Geometry: final body of the model. Coordinates: model frame, mm. Face numbers are marked on the shaded views. A direction names the side the tool comes from. Give positions to 0.01 mm unless a question says otherwise; leave off trailing zeros. Loops run counter-clockwise (first coordinate to the right, second up) from the corner with the lowest first, then second, coordinate; pieces in that order, holes last. Notation, with made-up numbers: M 76,69.25 L 84,69.25 A17 cw 84,88.25 Z; hole C 53,67 d5. An arc over 180 degrees is marked long. One line per question, with ' | ' between items. Start each with the question number.
from build123d import *

# Parameters (mm, degrees)
BOSS_EXTRUDE1_DEPTH            = 294.64
SKETCH3_W                      = 68.7
SKETCH3_H                      = 6.35
BOSS_EXTRUDE2_DEPTH            = 48
CUT_EXTRUDE2_REACH             = 304.363
SKETCH4_R                      = 1.3890625
SKETCH4_R_2                    = 11
SKETCH4_W                      = 26
SKETCH4_H                      = 72
CUT_EXTRUDE3_REACH             = 303.286
SKETCH5_R                      = 1.7859375
CUT_EXTRUDE4_REACH             = 309.814
SKETCH6_R                      = 1.3890625
CUT_EXTRUDE4_DIRECTION_2_REACH = 309.814
CUT_EXTRUDE5_REACH             = 309.814
SKETCH11_R                     = 0.889
SKETCH12_W                     = 68.7
SKETCH12_H                     = 6.35
CUT_EXTRUDE6_DEPTH             = 50.8
BOSS_EXTRUDE3_DEPTH            = 50
SKETCH14_W                     = 81.4
SKETCH14_H                     = 54.35
BOSS_EXTRUDE4_DEPTH            = 6.35
SKETCH15_W                     = 68.7
SKETCH15_H                     = 50
BOSS_EXTRUDE5_DEPTH            = 1
SKETCH16_W                     = 190.5
SKETCH16_H                     = 19.05
CUT_EXTRUDE7_DEPTH             = 4.175
SKETCH17_W                     = 190.5
SKETCH17_H                     = 19.05
CUT_EXTRUDE8_DEPTH             = 4.175
CUT_EXTRUDE9_DEPTH             = 310.015097083
CUT_EXTRUDE9_DEPTH_BACK        = 310.015097083
SKETCH18_R                     = 0.889


with BuildPart() as part:
    # Sketch1 → Boss-Extrude1 (new body)
    with BuildSketch(Plane.XY):
        Polygon((0, 0), (34.35, 0), (34.35, 48), (40.7, 48), (40.7, -6.35), (0, -6.35), align=None)
    extrude(amount=BOSS_EXTRUDE1_DEPTH)

    # Mirror1: part across plane


with BuildPart() as part_1:
    add(part.part)
    add(part.part.mirror(Plane(origin=(0, -6.35, 294.64), x_dir=(0, 0, 1), z_dir=(1, 0, 0))))

    # Sketch3 → Boss-Extrude2 (add)
    with BuildSketch(Plane(origin=(0, 0, 0), x_dir=(1, 0, 0), z_dir=(0, 1, 0))):
        with Locations((0, -3.175)):
            Rectangle(SKETCH3_W, SKETCH3_H)
    extrude(amount=BOSS_EXTRUDE2_DEPTH)

    # Sketch4 → Cut-Extrude2 (cut, up to next)
    with BuildSketch(Plane.XZ.offset(6.35), mode=Mode.PRIVATE) as cut_extrude2_sk1:
        with Locations((0, 12.7)):
            Circle(SKETCH4_R)
    cut_extrude2_tool1 = extrude(cut_extrude2_sk1.sketch, amount=-CUT_EXTRUDE2_REACH, mode=Mode.PRIVATE) & part_1.part
    # Sketch4 → Cut-Extrude2 (cut, up to next)
    with BuildSketch(Plane.XZ.offset(6.35), mode=Mode.PRIVATE) as cut_extrude2_sk2:
        with Locations((0, 95.2)):
            Circle(SKETCH4_R)
    cut_extrude2_tool2 = extrude(cut_extrude2_sk2.sketch, amount=-CUT_EXTRUDE2_REACH, mode=Mode.PRIVATE) & part_1.part
    # Sketch4 → Cut-Extrude2 (cut, up to next)
    with BuildSketch(Plane.XZ.offset(6.35), mode=Mode.PRIVATE) as cut_extrude2_sk3:
        with Locations((0, 53.95)):
            Circle(SKETCH4_R_2)
    cut_extrude2_tool3 = extrude(cut_extrude2_sk3.sketch, amount=-CUT_EXTRUDE2_REACH, mode=Mode.PRIVATE) & part_1.part
    # Sketch4 → Cut-Extrude2 (cut, up to next)
    with BuildSketch(Plane.XZ.offset(6.35), mode=Mode.PRIVATE) as cut_extrude2_sk4:
        with Locations((-3.2622, 160.64)):
            Rectangle(SKETCH4_W, SKETCH4_H)
    cut_extrude2_tool4 = extrude(cut_extrude2_sk4.sketch, amount=-CUT_EXTRUDE2_REACH, mode=Mode.PRIVATE) & part_1.part
    add(cut_extrude2_tool1.solids().sort_by_distance((0, -6.35, 12.7))[0], mode=Mode.SUBTRACT)
    add(cut_extrude2_tool2.solids().sort_by_distance((0, -6.35, 95.2))[0], mode=Mode.SUBTRACT)
    add(cut_extrude2_tool3.solids().sort_by_distance((0, -6.35, 53.95))[0], mode=Mode.SUBTRACT)
    add(cut_extrude2_tool4.solids().sort_by_distance((-3.2622, -6.35, 160.64))[0], mode=Mode.SUBTRACT)

    # Sketch5 → Cut-Extrude3 (cut, up to next)
    with BuildSketch(Plane(origin=(0, 0, 0), x_dir=(1, 0, 0), z_dir=(0, 1, 0)), mode=Mode.PRIVATE) as cut_extrude3_sk1:
        with Locations(Location((16.0628, -195.74, 0), (0, 0, 270))):
            Circle(SKETCH5_R)
    cut_extrude3_tool1 = extrude(cut_extrude3_sk1.sketch, amount=-CUT_EXTRUDE3_REACH, mode=Mode.PRIVATE) & part_1.part
    # Sketch5 → Cut-Extrude3 (cut, up to next)
    with BuildSketch(Plane(origin=(0, 0, 0), x_dir=(1, 0, 0), z_dir=(0, 1, 0)), mode=Mode.PRIVATE) as cut_extrude3_sk2:
        with Locations(Location((16.0628, -139.74, 0), (0, 0, 270))):
            Circle(SKETCH5_R)
    cut_extrude3_tool2 = extrude(cut_extrude3_sk2.sketch, amount=-CUT_EXTRUDE3_REACH, mode=Mode.PRIVATE) & part_1.part
    add(cut_extrude3_tool1.solids().sort_by_distance((16.0628, 0, 195.74))[0], mode=Mode.SUBTRACT)
    add(cut_extrude3_tool2.solids().sort_by_distance((16.0628, 0, 139.74))[0], mode=Mode.SUBTRACT)

    # Cut-Extrude4: up to this face of the body (flat: up to its plane)
    cut_extrude4_end = Plane(part_1.part.faces().sort_by_distance((40.7, 20.825, 147.32))[0])
    # Sketch6 → Cut-Extrude4 (cut, up to the picked face)
    with BuildSketch(Plane(origin=(-34.35, 0, 0), x_dir=(0, 0, -1), z_dir=(1, 0, 0)), mode=Mode.PRIVATE) as cut_extrude4_sk1:
        with Locations(Location((-287.14, 32.15, 0), (0, 0, 180))):
            Circle(SKETCH6_R)
    cut_extrude4_tool1 = split(extrude(cut_extrude4_sk1.sketch, amount=CUT_EXTRUDE4_REACH, mode=Mode.PRIVATE), bisect_by=cut_extrude4_end, keep=Keep.BOTH, mode=Mode.PRIVATE)
    # Sketch6 → Cut-Extrude4 (cut, up to the picked face)
    with BuildSketch(Plane(origin=(-34.35, 0, 0), x_dir=(0, 0, -1), z_dir=(1, 0, 0)), mode=Mode.PRIVATE) as cut_extrude4_sk2:
        with Locations(Location((-122.14, 32.15, 0), (0, 0, 180))):
            Circle(SKETCH6_R)
    cut_extrude4_tool2 = split(extrude(cut_extrude4_sk2.sketch, amount=CUT_EXTRUDE4_REACH, mode=Mode.PRIVATE), bisect_by=cut_extrude4_end, keep=Keep.BOTH, mode=Mode.PRIVATE)
    add(cut_extrude4_tool1.solids().sort_by(Axis((-34.35, 32.15, 287.14), (1, 0, 0)))[0], mode=Mode.SUBTRACT)
    add(cut_extrude4_tool2.solids().sort_by(Axis((-34.35, 32.15, 122.14), (1, 0, 0)))[0], mode=Mode.SUBTRACT)

    # Cut-Extrude4 direction 2: up to this face of the body (flat: up to its plane)
    cut_extrude4_direction_2_end = Plane(part_1.part.faces().sort_by_distance((-40.7, 20.825, 147.32))[0])
    # Sketch6 → Cut-Extrude4 direction 2 (cut, up to the picked face)
    with BuildSketch(Plane(origin=(-34.35, 0, 0), x_dir=(0, 0, -1), z_dir=(1, 0, 0)), mode=Mode.PRIVATE) as cut_extrude4_direction_2_sk1:
        with Locations(Location((-287.14, 32.15, 0), (0, 0, 180))):
            Circle(SKETCH6_R)
    cut_extrude4_direction_2_tool1 = split(extrude(cut_extrude4_direction_2_sk1.sketch, amount=-CUT_EXTRUDE4_DIRECTION_2_REACH, mode=Mode.PRIVATE), bisect_by=cut_extrude4_direction_2_end, keep=Keep.BOTH, mode=Mode.PRIVATE)
    # Sketch6 → Cut-Extrude4 direction 2 (cut, up to the picked face)
    with BuildSketch(Plane(origin=(-34.35, 0, 0), x_dir=(0, 0, -1), z_dir=(1, 0, 0)), mode=Mode.PRIVATE) as cut_extrude4_direction_2_sk2:
        with Locations(Location((-122.14, 32.15, 0), (0, 0, 180))):
            Circle(SKETCH6_R)
    cut_extrude4_direction_2_tool2 = split(extrude(cut_extrude4_direction_2_sk2.sketch, amount=-CUT_EXTRUDE4_DIRECTION_2_REACH, mode=Mode.PRIVATE), bisect_by=cut_extrude4_direction_2_end, keep=Keep.BOTH, mode=Mode.PRIVATE)
    add(cut_extrude4_direction_2_tool1.solids().sort_by(Axis((-34.35, 32.15, 287.14), (-1, 0, 0)))[0], mode=Mode.SUBTRACT)
    add(cut_extrude4_direction_2_tool2.solids().sort_by(Axis((-34.35, 32.15, 122.14), (-1, 0, 0)))[0], mode=Mode.SUBTRACT)

    # Sketch11 → Cut-Extrude5 (cut, up to next)
    with BuildSketch(Plane.ZY.offset(-34.35), mode=Mode.PRIVATE) as cut_extrude5_sk1:
        with Locations((13.75, 5.5)):
            Circle(SKETCH11_R)
    cut_extrude5_tool1 = extrude(cut_extrude5_sk1.sketch, amount=-CUT_EXTRUDE5_REACH, mode=Mode.PRIVATE) & part_1.part
    # Sketch11 → Cut-Extrude5 (cut, up to next)
    with BuildSketch(Plane.ZY.offset(-34.35), mode=Mode.PRIVATE) as cut_extrude5_sk2:
        with Locations((13.75, 15)):
            Circle(SKETCH11_R)
    cut_extrude5_tool2 = extrude(cut_extrude5_sk2.sketch, amount=-CUT_EXTRUDE5_REACH, mode=Mode.PRIVATE) & part_1.part
    # Sketch11 → Cut-Extrude5 (cut, up to next)
    with BuildSketch(Plane.ZY.offset(-34.35), mode=Mode.PRIVATE) as cut_extrude5_sk3:
        with Locations((140.81, 15)):
            Circle(SKETCH11_R)
    cut_extrude5_tool3 = extrude(cut_extrude5_sk3.sketch, amount=-CUT_EXTRUDE5_REACH, mode=Mode.PRIVATE) & part_1.part
    # Sketch11 → Cut-Extrude5 (cut, up to next)
    with BuildSketch(Plane.ZY.offset(-34.35), mode=Mode.PRIVATE) as cut_extrude5_sk4:
        with Locations((140.81, 5.5)):
            Circle(SKETCH11_R)
    cut_extrude5_tool4 = extrude(cut_extrude5_sk4.sketch, amount=-CUT_EXTRUDE5_REACH, mode=Mode.PRIVATE) & part_1.part
    add(cut_extrude5_tool1.solids().sort_by_distance((34.35, 5.5, 13.75))[0], mode=Mode.SUBTRACT)
    add(cut_extrude5_tool2.solids().sort_by_distance((34.35, 15, 13.75))[0], mode=Mode.SUBTRACT)
    add(cut_extrude5_tool3.solids().sort_by_distance((34.35, 15, 140.81))[0], mode=Mode.SUBTRACT)
    add(cut_extrude5_tool4.solids().sort_by_distance((34.35, 5.5, 140.81))[0], mode=Mode.SUBTRACT)

    # Sketch12 → Cut-Extrude6 (cut)
    with BuildSketch(Plane.XY.offset(294.64)):
        with Locations((0, -3.175)):
            Rectangle(SKETCH12_W, SKETCH12_H)
    extrude(amount=-CUT_EXTRUDE6_DEPTH, mode=Mode.SUBTRACT)

    # Sketch13 → Boss-Extrude3 (add)
    with BuildSketch(Plane(origin=(0, 0, 0), x_dir=(-1, 0, 0), z_dir=(0, 0, -1))):
        Polygon((34.35, 48), (34.35, 0), (-34.35, 0), (-34.35, 48), (-40.7, 48), (-40.7, -6.35), (40.7, -6.35), (40.7, 48), align=None)
    extrude(amount=BOSS_EXTRUDE3_DEPTH)

    # Sketch14 → Boss-Extrude4 (add)
    with BuildSketch(Plane(origin=(0, 0, -50), x_dir=(-1, 0, 0), z_dir=(0, 0, -1))):
        with Locations((0, 20.825)):
            Rectangle(SKETCH14_W, SKETCH14_H)
    extrude(amount=BOSS_EXTRUDE4_DEPTH)

    # Sketch15 → Boss-Extrude5 (add)
    with BuildSketch(Plane(origin=(0, 48, 0), x_dir=(1, 0, 0), z_dir=(0, 1, 0))):
        Polygon((40.7, -294.64), (40.7, 56.35), (-40.7, 56.35), (-40.7, -294.64), (-34.35, -294.64), (-34.35, -6.35), (34.35, -6.35), (34.35, -294.64), align=None)
        with Locations((0, 25)):
            Rectangle(SKETCH15_W, SKETCH15_H, mode=Mode.SUBTRACT)
    extrude(amount=BOSS_EXTRUDE5_DEPTH)

    # Sketch16 → Cut-Extrude7 (cut)
    with BuildSketch(Plane(origin=(-34.35, 0, 0), x_dir=(0, 0, -1), z_dir=(1, 0, 0))):
        with Locations((-199.39, 32.15)):
            Rectangle(SKETCH16_W, SKETCH16_H)
    extrude(amount=-CUT_EXTRUDE7_DEPTH, mode=Mode.SUBTRACT)

    # Sketch17 → Cut-Extrude8 (cut)
    with BuildSketch(Plane.ZY.offset(-34.35)):
        with Locations((199.39, 32.15)):
            Rectangle(SKETCH17_W, SKETCH17_H)
    extrude(amount=-CUT_EXTRUDE8_DEPTH, mode=Mode.SUBTRACT)

    # Sketch18 → Cut-Extrude9 (cut, two sides: drawn at the far end of the back side and taken through both)
    with BuildSketch(Plane(origin=(-38.525, 0, 0), x_dir=(0, 0, -1), z_dir=(1, 0, 0)).offset(-CUT_EXTRUDE9_DEPTH_BACK)):
        with Locations((-287.14, 39.77)):
            Circle(SKETCH18_R)
        with Locations((-287.14, 24.53)):
            Circle(SKETCH18_R)
        with Locations((-122.14, 39.77)):
            Circle(SKETCH18_R)
        with Locations((-122.14, 24.53)):
            Circle(SKETCH18_R)
    extrude(amount=CUT_EXTRUDE9_DEPTH + CUT_EXTRUDE9_DEPTH_BACK, mode=Mode.SUBTRACT)


solid = part_1.part
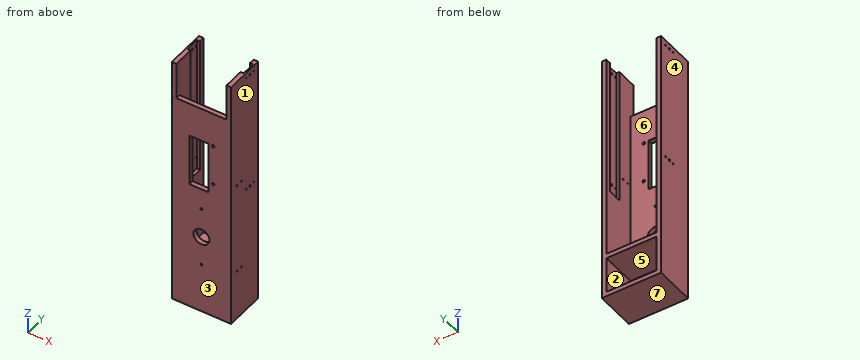
Q1. Section B-B, the plane x = -27.5. Output: boundary loops of the cut face in (y, z).
Q2. Material intervals for L1, parallel to Z at x = 16.5, y = -2; L2, parallel to Y at x = 36.25, z = 140.81 (3 decimals); L3, parallel to Z at x = 39.85, y = 24.53, sorted ascending.
Q3. Contact query for flat-ended pins moving along their axis: pin 1 (10 mm diameter, centred on x = -19.5, z = -13, fed in from +Y); pin 2 (1.1 mm diameter, centred on y = 39.77, z = 122.14, fed in from -X). Output: stop coordinate, or through.
Q4. Set-up query: the marked faces 5, 6 and 7. Return all of +Z, -Z, +X, -X, +Y, -Y with unobstructed straight access to the full face (end or side cutting, diameter ignored); none if empty.
Q5. Section A-A, the plane z = 187. Output: boundary loops of the cut face in (x, y) (3 decimals), plus the area to 3 significant figures.
Q6. Section D-D, the plane z = 53.95. Output: boundary loops of the cut face in (x, y).
Q7. Draft query along X for the marked faces 1, 2, 3 and 4. Return one class per face: released by +X, released by -X, zero draft, split by the parting line, or undercut.
Q8. Section C-C, the plane x = -5. Output: boundary loops of the cut face in (y, z), plus the area to 3 significant figures.
Model answer:
1) outline: M -6.35,-56.35 L 49,-56.35 L 49,-50 L 0,-50 L 0,0 L 49,0 L 49,6.35 L 0,6.35 L 0,243.84 L -6.35,243.84 Z
2) L1: z = -56.35 to 138.01, 141.47 to 194.01, 197.47 to 243.84 | L2: y = -6.35 to 4.611, 6.389 to 14.111, 15.889 to 22.625, 41.675 to 49 | L3: z = -56.35 to 121.25, 123.03 to 286.25, 288.03 to 294.64
3) pin 1: stops at y = 0 | pin 2: passes through
4) face 5: +Y | face 6: +Z, +Y | face 7: -Z, +X, -X, +Y, -Y
5) outline: M -40.7,-6.35 L -16.262,-6.35 L -16.262,0 L -34.35,0 L -34.35,22.625 L -38.525,22.625 L -38.525,41.675 L -34.35,41.675 L -34.35,49 L -40.7,49 Z; M 9.738,-6.35 L 40.7,-6.35 L 40.7,49 L 34.35,49 L 34.35,41.675 L 38.525,41.675 L 38.525,22.625 L 34.35,22.625 L 34.35,0 L 9.738,0 Z | area: 815 mm^2
6) outline: M -40.7,-6.35 L -11,-6.35 L -11,0 L -34.35,0 L -34.35,49 L -40.7,49 Z; M 11,-6.35 L 40.7,-6.35 L 40.7,49 L 34.35,49 L 34.35,0 L 11,0 Z
7) face 1: released by +X | face 2: undercut | face 3: zero draft | face 4: released by -X
8) outline: M -6.35,-56.35 L 49,-56.35 L 49,-50 L 0,-50 L 0,0 L 49,0 L 49,6.35 L 0,6.35 L 0,44.15 L -6.35,44.15 Z; M -6.35,63.75 L 0,63.75 L 0,124.64 L -6.35,124.64 Z; M -6.35,196.64 L 0,196.64 L 0,243.84 L -6.35,243.84 Z | area: 1,950 mm^2
